Here's the drawing with two shaded views (mm, measured from the low corner). I have some questions. A direction names the side the tool comes from. Round coordinates to 2 decimals unless told otherwise and drop trailing zeros. Order: outer loops, then holes, each group sorted by start corner. A loop starts at its lowest first (then second) coordinate and runs counter-clockwise, first axis right, second up. Notation, with made-up numbers: (21, -37) -> (36, -37) arc R28 cw to (36, -18) -> close; hole circle Ø7 at (-0.75, -37). An arc over 180 degrees is marked (long way). One line per question, with ' | ' between items.
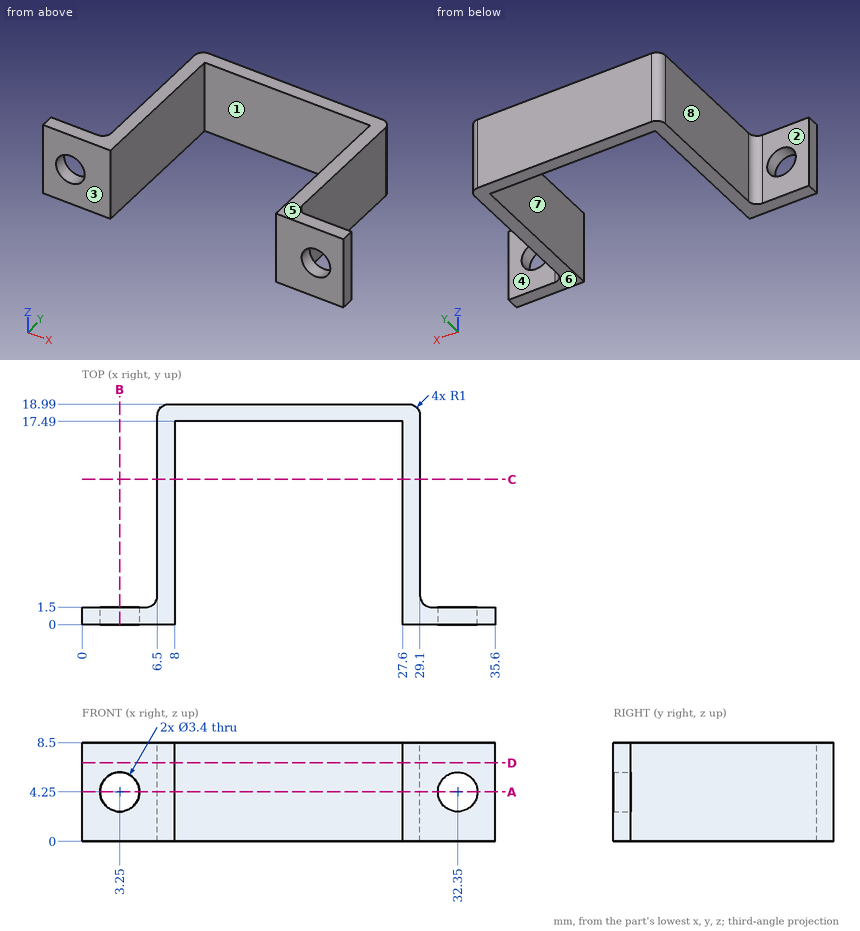
1. If we mould it in two halves opening along X, with no side actions, what happens to the marked faces 6, 7 and 8? For each: pulls with the +X half, pulls with the -X half, needs draft (parallel to the pull), parting line crosses it, or undercut.
From the geometry:
face 6: needs draft | face 7: undercut | face 8: pulls with the -X half
2. I want a section at D-D on z = 6.75. List the corners of the cut face in (x, y) for me, and give its area (3 significant figures).
From the geometry:
outline: (0, 0) -> (8, 0) -> (8, 17.49) -> (27.6, 17.49) -> (27.6, 0) -> (35.6, 0) -> (35.6, 1.5) -> (30.1, 1.5) arc R1 cw to (29.1, 2.5) -> (29.1, 17.99) arc R1 ccw to (28.1, 18.99) -> (7.5, 18.99) arc R1 ccw to (6.5, 17.99) -> (6.5, 2.5) arc R1 cw to (5.5, 1.5) -> (0, 1.5) -> close | area: 106 mm²
3. I need wall thicknesses on probe 1 along X at (y, z) = (12.75, 2.5); probe 2 along Z at (x, y) = (3.25, 0.95); probe 3 along Y at (x, z) = (13, 5.25). Which ranges of each line are inside material? Lowest first, please.
From the geometry:
probe 1: x = 6.5 to 8, 27.6 to 29.1 | probe 2: z = 0 to 2.55, 5.95 to 8.5 | probe 3: y = 17.49 to 18.99
4. On a 3-axis mill with a long thin cutter (end or side, diameter ignored), from which of +Z, -Z, +X, -X, +Y, -Y can I reach the whole of each face in a straight line? I mean the marked faces 1, 2, 3, 4 and 5. Say none if no direction works.
From the geometry:
face 1: +Z, -Z, -Y | face 2: +Z, -Z, -X, +Y | face 3: +Z, -Z, +X, -X, -Y | face 4: +Z, -Z, +X, +Y | face 5: +Z, +X, -X, +Y, -Y
5. I want a section at A-A on z = 4.25. List the corners of the cut face in (x, y) for me.
From the geometry:
outline: (0, 0) -> (1.55, 0) -> (1.55, 1.5) -> (0, 1.5) -> close; (4.95, 0) -> (8, 0) -> (8, 17.49) -> (27.6, 17.49) -> (27.6, 0) -> (30.65, 0) -> (30.65, 1.5) -> (30.1, 1.5) arc R1 cw to (29.1, 2.5) -> (29.1, 17.99) arc R1 ccw to (28.1, 18.99) -> (7.5, 18.99) arc R1 ccw to (6.5, 17.99) -> (6.5, 2.5) arc R1 cw to (5.5, 1.5) -> (4.95, 1.5) -> close; (34.05, 0) -> (35.6, 0) -> (35.6, 1.5) -> (34.05, 1.5) -> close
6. I'm going to push flat-ended pins straight in: pin 1 (4 mm diameter, centred on y = 6, z = 3, fed in from -X); pin 2 (2.5 mm diameter, centred on y = 8.5, z = 5, fed in from +X); pin 3 (1 mm diameter, centred on x = 19.5, z = 5, fed in from -Y); pin 4 (2.5 mm diameter, centred on x = 3.25, z = 4.25, fed in from +Y). Where does each tip first touch, or does it pass through?
From the geometry:
pin 1: stops at x = 6.5 | pin 2: stops at x = 29.1 | pin 3: stops at y = 17.49 | pin 4: passes through
7. I want a section at C-C on y = 12.5. List the corners of the cut face in (x, z) for me, and give its area (3 significant figures).
From the geometry:
outline: (6.5, 0) -> (8, 0) -> (8, 8.5) -> (6.5, 8.5) -> close; (27.6, 0) -> (29.1, 0) -> (29.1, 8.5) -> (27.6, 8.5) -> close | area: 25.5 mm²
8. I want a section at B-B on x = 3.25. List the corners of the cut face in (y, z) for me.
From the geometry:
outline: (0, 0) -> (1.5, 0) -> (1.5, 2.55) -> (0, 2.55) -> close; (0, 5.95) -> (1.5, 5.95) -> (1.5, 8.5) -> (0, 8.5) -> close
